Check sheet for the modelled part. Datum: model origin and axes. Units: mm. Round coordinates to 2 decimals unless told otherwise and drop trailing zeros. Loops run counter-clockwise (first coordinate to the right, second up) from the corner with the lowest first, then second, coordinate; pieces in that order, holes last. Notation, with made-up numbers: (30.25, -38) - (71.25, -38) arc R26 cw to (71.25, -1) - close; hole circle Ø10 at (87.25, 28). An arc over 180 degrees is marked (long way). Return JSON: item names as keys, results as strings.
Autodesk Inventor part; units mm, degrees
ref_plane "YZ Plane" through (0, 0, 0) normal (1, 0, 0) x (0, 1, 0)
ref_plane "XZ Plane" through (0, 0, 0) normal (0, 1, 0) x (-1, 0, 0)
ref_plane "XY Plane" through (0, 0, 0) normal (0, 0, 1) x (1, 0, 0)
sketch "Sketch1" plane through (0, 0, 0) normal (0, 0, 1) x (1, 0, 0)
  line L0 (0, 0) -> (8, 0) construction
  line L1 (0, -2.5) -> (8, -2.5)
  line L2 (8, 2.5) -> (0, 2.5)
  arc A0 (0, 2.5) -> (0, -2.5) centre (0, 0) ccw
  arc A1 (8, -2.5) -> (8, 2.5) centre (8, 0) ccw
  circle A2 centre (8, 0) radius 1.5
  circle A3 centre (0, 0) radius 1.5
  point P0 (4, 0)
  dimension "d0" = 8
  dimension "d1" = 5
  dimension "d2" = 3
  dimension "d3" = 3
extrude "Extrusion1" add sketch "Sketch1" along normal mid plane 1
properties part number "CompressionRollerActuatorLinkage1" material "Stainless Steel"
Q1. Scan lines: probe 1 along Y at (x, z) = (0, -0.15); probe 2 along X at (y, z) = (-1.15, -0.3); probe 3 along X at (y, z) = (0.85, -0.1). Record each from-to range of solid material in increasing order. Write a range as [from, to].
Answer key:
{"probe 1": "y = [-2.5, -1.5], [1.5, 2.5]", "probe 2": "x = [-2.22, -0.96], [0.96, 7.04], [8.96, 10.22]", "probe 3": "x = [-2.35, -1.24], [1.24, 6.76], [9.24, 10.35]"}
Q2. Draft check along X on faces 1 (the face through (4, 0, -0.5)), 2 (the face through (-2.5, -0.1, 0)), 3 (the face through (-1.5, -0.07, -0.01)). Enter one of: released by +X, released by -X, zero draft, split by the parting line, or undercut.
Answer key:
{"face 1": "zero draft", "face 2": "released by -X", "face 3": "undercut"}
Q3. Sectioned sample at B-B (z = -0.25). Enter the section's corners in (x, y).
Answer key:
{"outline": "(0, -2.5) - (8, -2.5) arc R2.5 ccw to (8, 2.5) - (0, 2.5) arc R2.5 ccw to start; hole circle Ø3 at (0, 0); hole circle Ø3 at (8, 0)"}
Q4. Sectioned sample at D-D (y = 1.65). Enter the section's corners in (x, z), plus the area to 3 significant figures.
Answer key:
{"outline": "(-1.88, -0.5) - (9.88, -0.5) - (9.88, 0.5) - (-1.88, 0.5) - close", "area": "11.8 mm²"}
Q5. Sectioned sample at C-C (y = 0.95). Enter the section's corners in (x, z).
Answer key:
{"outline": "(-2.31, -0.5) - (-1.16, -0.5) - (-1.16, 0.5) - (-2.31, 0.5) - close; (1.16, -0.5) - (6.84, -0.5) - (6.84, 0.5) - (1.16, 0.5) - close; (9.16, -0.5) - (10.31, -0.5) - (10.31, 0.5) - (9.16, 0.5) - close"}
Q6. Sectioned sample at A-A (y = 0). Enter the section's corners in (x, z).
Answer key:
{"outline": "(-2.5, -0.5) - (-1.5, -0.5) - (-1.5, 0.5) - (-2.5, 0.5) - close; (1.5, -0.5) - (6.5, -0.5) - (6.5, 0.5) - (1.5, 0.5) - close; (9.5, -0.5) - (10.5, -0.5) - (10.5, 0.5) - (9.5, 0.5) - close"}
